Here's how the part is built. I have some questions about the finished solid (model axes, mm). Face numbers are marked on the shaded views. A direction names the side the tool comes from. Give positions to 0.01 mm unless a question says otherwise; leave off trailing zeros. Loops run counter-clockwise (first coordinate to the right, second up) from the corner with the lowest first, then second, coordinate; pieces in that order, holes last.
Q1. Suppose I cut it at C-C (x = 6). List the corners of the cut face in (y, z) for me, and give its area (4 significant figures).
Q2. For the marked faces 4 and 5, which set-ups out of +Z, -Z, +X, -X, +Y, -Y let a thin tool reach every point of the face, with its end or its side?
Q3. Suppose I cut it at B-B (z = -37.5). List the corners of the cut face in (x, y) for me, and give its area (3 significant figures).
Q4. I'm going to push flat-ended pins straight in: P1, Ø2.5, axis at x = 46, z = -45.5, coming from the +Y side; P2, Ø1.9, axis at x = 18.5, z = -0.5, coming from the -Y side; P3, Ø6.5, axis at x = -36.5, z = -39, coming from the +Y side. Where does each tip first touch, or does it pass through?
Q5. Thinking about a two-plate mould opening in Z: for the marked faces 1, 2 and 3, which applies, pulls with the +Z half, pulls with the -Z half, needs draft (parallel to the pull), parting line crosses it, or undercut?
Q6. Suppose I cut it at D-D (z = 3.5). List the corners of the cut face in (x, y) for me.
Q7. Suppose I cut it at A-A (y = 9.5). List the corners of the cut face in (x, z) for me, and give its area (3 significant figures).
Q8. I need wall thicknesses on probe 1 along X at (y, z) = (18.6, 0); probe 2 along Z at (x, y) = (40, 12). Which ranges of each line are inside material? Lowest first, please.
```python
from build123d import *

# Parameters (mm, degrees)
SKETCH2_W           = 115
SKETCH2_H           = 115
BOSS_EXTRUDE1_DEPTH = 35
SHELL1_T            = -2.5
SKETCH3_R           = 4.5
BOSS_EXTRUDE4_DEPTH = 28
FILLET1_R           = 1.5
FILLET2_R           = 1.5
FILLET3_R           = 1.5
FILLET4_R           = 1.5
SKETCH4_W           = 65
SKETCH4_H           = 65
CUT_EXTRUDE1_DEPTH  = 89.529656048
SKETCH5_W           = 8
SKETCH5_H           = 112
BOSS_EXTRUDE5_DEPTH = 4
SKETCH7_R           = 0.85
CUT_EXTRUDE10_DEPTH = 3
SKETCH15_R          = 3
BOSS_EXTRUDE6_DEPTH = 4


with BuildPart() as part:
    # Sketch2 → Boss-Extrude1 (new body)
    with BuildSketch(Plane(origin=(0, 0, 0), x_dir=(1, 0, 0), z_dir=(0, 1, 0))):
        Rectangle(SKETCH2_W, SKETCH2_H)
    extrude(amount=BOSS_EXTRUDE1_DEPTH)

    # Shell1
    shell1_openings = [part.faces().sort_by_distance(p)[0] for p in [
        (0, 35, 0),
    ]]
    offset(amount=SHELL1_T, openings=shell1_openings, kind=Kind.INTERSECTION)

    # Sketch3 → Boss-Extrude4 (add)
    with BuildSketch(Plane(origin=(0, 2.5, 0), x_dir=(1, 0, 0), z_dir=(0, 1, 0))):
        with Locations(Location((-45.72, -45.53, 0), (0, 0, 270))):
            Circle(SKETCH3_R)
        with Locations(Location((-45.72, 45.53, 0), (0, 0, 270))):
            Circle(SKETCH3_R)
        with Locations(Location((45.72, 45.53, 0), (0, 0, 270))):
            Circle(SKETCH3_R)
        with Locations(Location((45.72, -45.53, 0), (0, 0, 270))):
            Circle(SKETCH3_R)
    extrude(amount=BOSS_EXTRUDE4_DEPTH)

    # Fillet1
    fillet1_edges = [part.edges().sort_by_distance(p)[0] for p in [
        (-45.72, 2.5, 41.03),
    ]]
    fillet(fillet1_edges, radius=FILLET1_R)

    # Fillet2
    fillet2_edges = [part.edges().sort_by_distance(p)[0] for p in [
        (-45.72, 2.5, -50.03),
    ]]
    fillet(fillet2_edges, radius=FILLET2_R)

    # Fillet3
    fillet3_edges = [part.edges().sort_by_distance(p)[0] for p in [
        (45.72, 2.5, -50.03),
    ]]
    fillet(fillet3_edges, radius=FILLET3_R)

    # Fillet4
    fillet4_edges = [part.edges().sort_by_distance(p)[0] for p in [
        (45.72, 2.5, 41.03),
    ]]
    fillet(fillet4_edges, radius=FILLET4_R)

    # Sketch4 → Cut-Extrude1 (cut, through all)
    with BuildSketch(Plane.XZ):
        Rectangle(SKETCH4_W, SKETCH4_H)
    extrude(amount=-CUT_EXTRUDE1_DEPTH, mode=Mode.SUBTRACT)

    # Sketch5 → Boss-Extrude5 (add)
    with BuildSketch(Plane(origin=(0, 17, 0), x_dir=(1, 0, 0), z_dir=(0, 1, 0))):
        with Locations((-18.5, 0)):
            Rectangle(SKETCH5_W, SKETCH5_H)
        with Locations((18.5, -0.001)):
            Rectangle(SKETCH5_W, SKETCH5_H)
    extrude(amount=BOSS_EXTRUDE5_DEPTH)

    # Sketch7 → Cut-Extrude10 (cut)
    with BuildSketch(Plane.XZ.offset(-17)):
        with Locations(Location((-18.5, 0, 0), (0, 0, 270))):
            Circle(SKETCH7_R)
        with Locations(Location((18.5, 0, 0), (0, 0, 270))):
            Circle(SKETCH7_R)
    extrude(amount=-CUT_EXTRUDE10_DEPTH, mode=Mode.SUBTRACT)

    # Sketch15 → Boss-Extrude6 (add)
    with BuildSketch(Plane.XZ):
        with Locations(Location((37.5, -37.5, 0), (0, 0, 270))):
            Circle(SKETCH15_R)
        with Locations(Location((-37.5, -37.5, 0), (0, 0, 270))):
            Circle(SKETCH15_R)
        with Locations(Location((-37.5, 37.5, 0), (0, 0, 270))):
            Circle(SKETCH15_R)
        with Locations(Location((37.5, 37.5, 0), (0, 0, 270))):
            Circle(SKETCH15_R)
    extrude(amount=-BOSS_EXTRUDE6_DEPTH)


solid = part.part
```
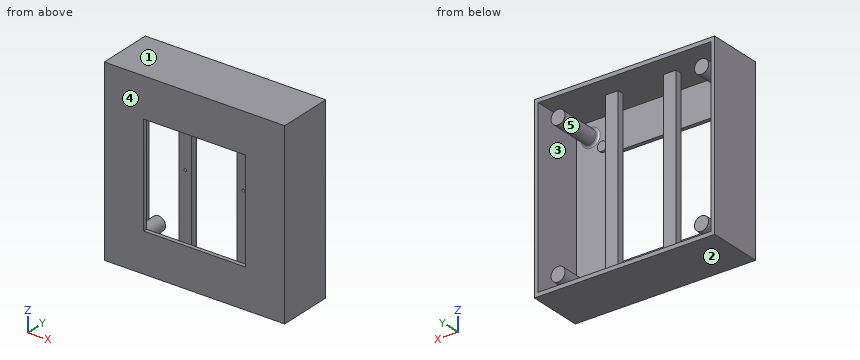
Solutions:
1. outline: (0, -57.5) - (35, -57.5) - (35, -55) - (2.5, -55) - (2.5, -32.5) - (0, -32.5) - close; (0, 32.5) - (2.5, 32.5) - (2.5, 55) - (35, 55) - (35, 57.5) - (0, 57.5) - close
1. area: 287.5 mm2
2. face 4: +Z, -Z, +X, -X, -Y
2. face 5: +Y
3. outline: (-57.5, 0) - (57.5, 0) - (57.5, 35) - (55, 35) - (55, 2.5) - (40.5, 2.5) - (40.5, 4) - (34.5, 4) - (34.5, 2.5) - (-34.5, 2.5) - (-34.5, 4) - (-40.5, 4) - (-40.5, 2.5) - (-55, 2.5) - (-55, 35) - (-57.5, 35) - close; (-22.5, 17) - (-14.5, 17) - (-14.5, 21) - (-22.5, 21) - close; (14.5, 17) - (22.5, 17) - (22.5, 21) - (14.5, 21) - close
3. area: 532 mm2
4. P1: stops at y = 30.5
4. P2: stops at y = 17
4. P3: stops at y = 4
5. face 1: pulls with the +Z half
5. face 2: pulls with the -Z half
5. face 3: undercut
6. outline: (-57.5, 0) - (-32.5, 0) - (-32.5, 2.5) - (-55, 2.5) - (-55, 35) - (-57.5, 35) - close; (-22.5, 17) - (-14.5, 17) - (-14.5, 21) - (-22.5, 21) - close; (14.5, 17) - (22.5, 17) - (22.5, 21) - (14.5, 21) - close; (32.5, 0) - (57.5, 0) - (57.5, 35) - (55, 35) - (55, 2.5) - (32.5, 2.5) - close
7. outline: (-57.5, -57.5) - (57.5, -57.5) - (57.5, 57.5) - (-57.5, 57.5) - close; circle Ø9 at (-45.72, -45.53); circle Ø9 at (-45.72, 45.53); circle Ø9 at (45.72, -45.53); circle Ø9 at (45.72, 45.53); hole (-55, -55) - (55, -55) - (55, 55) - (-55, 55) - close
7. area: 1,380 mm2
8. probe 1: x = -57.5 to -55, -22.5 to -19.35, -17.65 to -14.5, 14.5 to 17.65, 19.35 to 22.5, 55 to 57.5
8. probe 2: z = -57.5 to -55, 55 to 57.5
